```python
from build123d import *

# Parameters (mm, degrees)
SKETCH1_R           = 1
BOSS_EXTRUDE1_DEPTH = 25
SKETCH2_R           = 1.25
BOSS_EXTRUDE2_DEPTH = 1
FILLET1_R           = 1
BOSS_EXTRUDE5_START = 26
SKETCH3_R           = 1.25
BOSS_EXTRUDE5_DEPTH = 1
FILLET2_R           = 1


with BuildPart() as part:
    # Sketch1 → Boss-Extrude1 (new body)
    with BuildSketch(Plane(origin=(0, 0, 0), x_dir=(1, 0, 0), z_dir=(0, 1, 0))):
        with Locations(Location((0, 0, 0), (0, 0, 270))):
            Circle(SKETCH1_R)
    extrude(amount=BOSS_EXTRUDE1_DEPTH)

    # Sketch2 → Boss-Extrude2 (add)
    with BuildSketch(Plane(origin=(0, 0, 0), x_dir=(1, 0, 0), z_dir=(0, 1, 0))):
        with Locations(Location((0, 0, 0), (0, 0, 270))):
            Circle(SKETCH2_R)
    extrude(amount=-BOSS_EXTRUDE2_DEPTH)

    # Fillet1
    fillet1_edges = [part.edges().sort_by_distance(p)[0] for p in [
        (0, -1, -1.25),
    ]]
    fillet(fillet1_edges, radius=FILLET1_R - 0.0001)  # a hair under: the kernel refuses the full size

    # Sketch3 → Boss-Extrude5 (add)
    with BuildSketch(Plane(origin=(0, 0, 0), x_dir=(1, 0, 0), z_dir=(0, 1, 0)).offset(BOSS_EXTRUDE5_START)):
        with Locations(Location((0, 0, 0), (0, 0, 270))):
            Circle(SKETCH3_R)
    extrude(amount=-BOSS_EXTRUDE5_DEPTH)

    # Fillet2
    fillet2_edges = [part.edges().sort_by_distance(p)[0] for p in [
        (0, 26, -1.25),
    ]]
    fillet(fillet2_edges, radius=FILLET2_R - 0.0001)  # a hair under: the kernel refuses the full size


solid = part.part
```
Geometry: final body of the model. Coordinates: model frame, mm. Round coordinates to 2 decimals unless told otherwise and drop trailing zeros. Loops run counter-clockwise (first coordinate to the right, second up) from the corner with the lowest first, then second, coordinate; pieces in that order, holes last. Notation, with made-up numbers: (-2, -9) -> (31, -9) arc R24 ccw to (31, 23) -> close; hole circle Ø8 at (20, 23). An arc over 180 degrees is marked (long way). Use one line per item in the form item = value.
Item 1: Material intervals for probe 1 along Z at (x, y) = (-0.1, 22); probe 2 along X at (y, z) = (5.25, -0.05); probe 3 along Y at (x, z) = (-0.6, -0.95), sorted ascending.
Evaluation:
probe_1 = -0.99 to 0.99
probe_2 = -1 to 1
probe_3 = -0.49 to 0, 25 to 25.49
Item 2: Cut plane A-A on y = 14.25. Output: boundary loops of the cut face in (x, z), then the cut area to 3 significant figures.
Evaluation:
outline = circle Ø2 at (0, 0)
area = 3.14 mm2
Item 3: Contact query for a flat-ended pin moving along its axis: pin 1 Ø1.5 at (y, z) = (6, 0) entering from +X. Output: stop coordinate, or through.
Evaluation:
pin_1 = 1
